Input: part model. Units: mm. Frame: model coordinates. A direction names the side the tool comes from. Round coordinates to 2 decimals unless told otherwise and drop trailing zeros. Order: outer loops, then holes, each group sorted by start corner. A loop starts at its lowest first (then second) coordinate and runs counter-clockwise, first axis right, second up. Notation, with made-up numbers: (16.25, 26.25) - (72.25, 26.25) arc R21 cw to (72.25, 39.25) - close; hole circle Ø3 at (12.5, 81.25). An arc over 180 degrees is marked (long way). One line per item, written item: value. Start each with the question number.
from build123d import *

# Parameters (mm, degrees)
SKETCH1_R           = 25
BOSS_EXTRUDE1_DEPTH = 3
SKETCH3_R           = 6
SKETCH3_R_2         = 1
CUT_EXTRUDE1_DEPTH  = 36.482389998
SKETCH4_R           = 1
CUT_EXTRUDE2_DEPTH  = 36.482389998
CHAMFER1_SIZE       = 1
SKETCH5_R           = 18
CUT_EXTRUDE3_DEPTH  = 2


with BuildPart() as part:
    # Sketch1 → Boss-Extrude1 (new body)
    with BuildSketch(Plane(origin=(0, 0, 0), x_dir=(1, 0, 0), z_dir=(0, 1, 0))):
        with Locations(Location((0, 0, 0), (0, 0, 270))):
            Circle(SKETCH1_R)
    extrude(amount=BOSS_EXTRUDE1_DEPTH)

    # Sketch3 → Cut-Extrude1 (cut, through all)
    with BuildSketch(Plane(origin=(0, 3, 0), x_dir=(1, 0, 0), z_dir=(0, 1, 0))):
        with Locations(Location((0, 0, 0), (0, 0, 270))):
            Circle(SKETCH3_R)
        with Locations(Location((0, 7.5, 0), (0, 0, 270))):
            Circle(SKETCH3_R_2)
        with Locations(Location((0, -7.5, 0), (0, 0, 270))):
            Circle(SKETCH3_R_2)
    extrude(amount=-CUT_EXTRUDE1_DEPTH, mode=Mode.SUBTRACT)

    # Sketch4 → Cut-Extrude2 (cut, through all)
    with BuildSketch(Plane(origin=(0, 3, 0), x_dir=(1, 0, 0), z_dir=(0, 1, 0))):
        with Locations(Location((-15, 15, 0), (0, 0, 270))):
            Circle(SKETCH4_R)
        with Locations(Location((15, 15, 0), (0, 0, 270))):
            Circle(SKETCH4_R)
        with Locations(Location((15, -15, 0), (0, 0, 270))):
            Circle(SKETCH4_R)
        with Locations(Location((-15, -15, 0), (0, 0, 270))):
            Circle(SKETCH4_R)
    extrude(amount=-CUT_EXTRUDE2_DEPTH, mode=Mode.SUBTRACT)

    # Chamfer1
    chamfer1_edges = [part.edges().sort_by_distance(p)[0] for p in [
        (-15, 0, 14),
        (15, 0, 14),
        (15, 0, -16),
        (-15, 0, -16),
    ]]
    chamfer(chamfer1_edges, length=CHAMFER1_SIZE)

    # Sketch5 → Cut-Extrude3 (cut)
    with BuildSketch(Plane(origin=(0, 3, 0), x_dir=(1, 0, 0), z_dir=(0, 1, 0))):
        with Locations(Location((0, 0, 0), (0, 0, 270))):
            Circle(SKETCH5_R)
    extrude(amount=-CUT_EXTRUDE3_DEPTH, mode=Mode.SUBTRACT)


solid = part.part
Item 1: Section query A-A on z = 0. Return loops of the section in (x, y), and give its area (3 significant figures).
Item 2: Pull-direction query (X, two-part tool) for faces 1 (the face through (7.509, 1.479, 23.846)), 2 (the face through (-11, 3, 16)), 3 (the face through (14, 2, -15)); classes: released by +X, released by -X, zero draft, split by the parting line, or undercut.
Item 3: Section query B-B on z = 15. Return loops of the section in (x, y), and give its area (3 significant figures).
Item 4: Reachability of faces 4 (the face through (1.802, 0.507, 5.723)), 5 (the face through (-8, 1, 0)) from +Z, -Z, +X, -X, +Y, -Y: full face, straight path, thin tool, end or side. Return the list, or none.
Item 5: Line query: L1, parallel to X at y = 2.15, z = -15; L2, parallel to X at y = 2.2, z = 0; L3, parallel to Y at x = 9, z = -14.5. Output: solid intervals per line, ascending.
Item 6: Section query D-D on y = 1.55. Return loops of the section in (x, z), and give its area (3 significant figures).
Item 7: Section query C-C on x = 2. Return loops of the section in (y, z).
Item 8: First-contact query: pin 1 Ø1.6 at (x, z) = (15, 15) entering from -Y; pin 2 Ø1 at (y, z) = (1.5, -9) entering from +X; pin 3 Ø2.5 at (x, z) = (0, -7.5) entering from +Y; pin 4 Ø1 at (y, z) = (1, 19.5) entering from -X. Flat tips, straight axial feed; report the tip coordinate or a pass-through.
Geometry results:
1. outline: (-25, 0) - (-6, 0) - (-6, 1) - (-18, 1) - (-18, 3) - (-25, 3) - close; (6, 0) - (25, 0) - (25, 3) - (18, 3) - (18, 1) - (6, 1) - close
1. area: 66.0 mm^2
2. face 1: split by the parting line
2. face 2: zero draft
2. face 3: undercut
3. outline: (-20, 0) - (-17, 0) - (-16, 1) - (-16, 3) - (-20, 3) - close; (-14, 1) - (-13, 0) - (13, 0) - (14, 1) - (14, 3) - (9.95, 3) - (9.95, 1) - (-9.95, 1) - (-9.95, 3) - (-14, 3) - close; (16, 1) - (17, 0) - (20, 0) - (20, 3) - (16, 3) - close
3. area: 66.2 mm^2
4. face 4: +Y, -Y
4. face 5: +Y
5. L1: x = -20 to -16, -14 to -9.95, 9.95 to 14, 16 to 20
5. L2: x = -25 to -18, 18 to 25
5. L3: y = 0 to 1
6. outline: circle Ø50 at (0, 0); hole circle Ø36 at (0, 0); hole circle Ø2 at (-15, -15); hole circle Ø2 at (-15, 15); hole circle Ø2 at (15, -15); hole circle Ø2 at (15, 15)
6. area: 933 mm^2
7. outline: (0, -24.92) - (3, -24.92) - (3, -17.89) - (1, -17.89) - (1, -5.66) - (0, -5.66) - close; (0, 5.66) - (1, 5.66) - (1, 17.89) - (3, 17.89) - (3, 24.92) - (0, 24.92) - close
8. pin 1: passes through
8. pin 2: stops at x = 23.51
8. pin 3: stops at y = 1
8. pin 4: stops at x = -16.25
